```python
from build123d import *

# Parameters (mm, degrees)
BOSS_EXTRUDE6_START     = 1.5
BOSS_EXTRUDE6_DEPTH     = 1.5
BOSS_EXTRUDE7_START     = 3
SKETCH1_5_W             = 11.9
SKETCH1_5_H             = 5.3
SKETCH1_5_W_2           = 1.5
SKETCH1_5_H_2           = 5.936611654
BOSS_EXTRUDE7_DEPTH     = 7.93
BOSS_EXTRUDE8_START     = 10.93
BOSS_EXTRUDE8_OUTLINE_W = 11.9
BOSS_EXTRUDE8_OUTLINE_H = 12.736611654
BOSS_EXTRUDE8_DEPTH     = 0.75
SKETCH4_R               = 1.5
BOSS_EXTRUDE10_DEPTH    = 2.5


# Read off the part's stored shape, not the designer's step: Boss-Extrude8
with BuildPart() as part:
    # Sketch1 → Boss-Extrude6 (new body)
    with BuildSketch(Plane.ZY.offset(94.76563723).offset(BOSS_EXTRUDE6_START)):
        with BuildLine():
            Line((-51.759425025, -53.863488773), (-52.289755114, -53.333158684))
            ThreePointArc((-52.289755114, -53.333158684), (-52.343100233, -53.254101332), (-52.362978418, -53.160824194))
            Line((-52.362978418, -53.160824194), (-52.362978418, -48.300100424))
            Line((-52.362978418, -48.300100424), (-54.862978418, -48.300100424))
            Line((-54.862978418, -48.300100424), (-54.862978418, -61.036712078))
            Line((-54.862978418, -61.036712078), (-42.962978418, -61.036712078))
            Line((-42.962978418, -61.036712078), (-42.962978418, -48.300100424))
            Line((-42.962978418, -48.300100424), (-45.462978418, -48.300100424))
            Line((-45.462978418, -48.300100424), (-45.462978418, -53.156381989))
            ThreePointArc((-45.462978418, -53.156381989), (-45.482008535, -53.252052847), (-45.536201723, -53.333158684))
            Line((-45.536201723, -53.333158684), (-46.066531809, -53.86348877))
            ThreePointArc((-46.066531809, -53.86348877), (-46.147637646, -53.917681958), (-46.243308504, -53.936712075))
            Line((-46.243308504, -53.936712075), (-51.582648329, -53.936712078))
            ThreePointArc((-51.582648329, -53.936712078), (-51.678319187, -53.917681961), (-51.759425025, -53.863488773))
        make_face()
    extrude(amount=BOSS_EXTRUDE6_DEPTH)

    # Sketch1<5> → Boss-Extrude7 (add)
    with BuildSketch(Plane.ZY.offset(94.76563723).offset(BOSS_EXTRUDE7_START)):
        with Locations((-48.912978418, -58.386712078)):
            Rectangle(SKETCH1_5_W, SKETCH1_5_H)
        Polygon((-53.362978418, -55.636712078), (-53.362978418, -54.236712078), (-54.862978418, -54.236712078), (-54.862978418, -55.736712078), (-42.962978418, -55.736712078), (-42.962978418, -54.236712078), (-44.462978418, -54.236712078), (-44.462978418, -55.636712078), align=None)
        with Locations((-54.112978418, -51.268406251)):
            Rectangle(SKETCH1_5_W_2, SKETCH1_5_H_2)
        with Locations((-43.712978418, -51.268406251)):
            Rectangle(SKETCH1_5_W_2, SKETCH1_5_H_2)
    extrude(amount=BOSS_EXTRUDE7_DEPTH)

    # Boss-Extrude8 outline → Boss-Extrude8 (add)
    with BuildSketch(Plane.ZY.offset(94.76563723).offset(BOSS_EXTRUDE8_START)):
        with Locations((-48.912978418, -54.668406251)):
            Rectangle(BOSS_EXTRUDE8_OUTLINE_W, BOSS_EXTRUDE8_OUTLINE_H)
    extrude(amount=BOSS_EXTRUDE8_DEPTH)

    # Sketch4 → Boss-Extrude10 (add)
    # profile 1 of 2: a face of its own
    with BuildSketch(Plane.XZ.offset(61.036712078)):
        with BuildLine():
            Line((-102.26563723, -39.962978418), (-102.26563723, -42.962978418))
            Line((-102.26563723, -42.962978418), (-96.26563723, -42.962978418))
            Line((-96.26563723, -42.962978418), (-96.26563723, -39.962978418))
            ThreePointArc((-96.26563723, -39.962978418), (-99.26563723, -36.962978418), (-102.26563723, -39.962978418))
        make_face()
        with Locations(Location((-99.26563723, -39.962978418, 0), (0, 0, 270))):
            Circle(SKETCH4_R, mode=Mode.SUBTRACT)
    # profile 2 of 2: a face of its own
    with BuildSketch(Plane.XZ.offset(61.036712078)):
        with BuildLine():
            Line((-96.26563723, -57.862978418), (-96.26563723, -54.862978418))
            Line((-96.26563723, -54.862978418), (-102.26563723, -54.862978418))
            Line((-102.26563723, -54.862978418), (-102.26563723, -57.862978418))
            ThreePointArc((-102.26563723, -57.862978418), (-99.26563723, -60.862978418), (-96.26563723, -57.862978418))
        make_face()
        with Locations(Location((-99.26563723, -57.862978418, 0), (0, 0, 270))):
            Circle(SKETCH4_R, mode=Mode.SUBTRACT)
    extrude(amount=-BOSS_EXTRUDE10_DEPTH)


solid = part.part
```
For this review, take the finished solid that the model builds, in its own axes (mm). A direction names the side the tool comes from. Give positions to 0.01 mm unless a question says otherwise; leave off trailing zeros. Write each loop counter-clockwise with the first axis right and the second up, starting at its lowest first coordinate (ties: lowest second). Pieces come first, ordered by that corner, then holes.
Item 1: Take a section at B-B (x = -103.75). Give the boundary of the cut face in (y, z), and give its area (3 significant figures).
Item 2: Insertion check: P1, Ø2, axis at x = -101, y = -51.5, coming from the -Z side; P2, Ø3.5, axis at x = -100, y = -51.5, coming from the +Z side; P3, Ø1.6, axis at x = -97, z = -49, coming from the +Y side; P4, Ø1.8, axis at x = -99.27, z = -57.86, coming from the +Y side. Each pin has a flat end and moves straight along its axis. Give the tip position at first contact, or say it passes through.
Item 3: Wall thickness on probe 1 along Z at (x, y) = (-102.25, -54); probe 2 along X at (y, z) = (-49.25, -45.25); probe 3 along Y at (x, z) = (-101.5, -50.25): over which ranges is each line inside the solid? List them lowest first.
Item 4: Take a section at D-D (z = -59). Give the boundary of the cut face in (x, y), and give its area (3 significant figures).
Item 5: Take a section at C-C (y = -55). Give the boundary of the cut face in (x, z), and give its area (3 significant figures).
Item 6: The part is to be moulded in two halves that separate along X. For faces 1 (the face through (-101, -55, -42.963)), 2 (the face through (-99.84, -59.8, -41.35)), 3 (the face through (-106.446, -55, -49)), say which applies: +X half, -X half, draft (parallel to the pull), parting line (faces both ways), or undercut.
Item 7: Take a section at A-A (z = -48). Give the boundary of the cut face in (x, y).
Item 8: Machinability: for faces 4 (the face through (-102.266, -60, -41)), 5 (the face through (-102, -52, -53.363)), 6 (the face through (-97, -51, -52.363)), 7 (the face through (-100, -58.537, -56)), which of the approach directions +Z, -Z, +X, -X, +Y, -Y give a long, thin tool a straight path to every point of the face, cutting with its end or side? Answer none if there is none.
Established:
1. outline: (-61.04, -54.86) - (-48.3, -54.86) - (-48.3, -53.36) - (-55.64, -53.36) - (-55.64, -44.46) - (-48.3, -44.46) - (-48.3, -42.96) - (-61.04, -42.96) - close
1. area: 86.3 mm2
2. P1: stops at z = -54.86
2. P2: stops at z = -42.96
2. P3: stops at y = -53.94
2. P4: passes through
3. probe 1: z = -54.86 to -53.36, -44.46 to -42.96
3. probe 2: x = -106.45 to -105.7, -97.77 to -96.27
3. probe 3: y = -61.04 to -55.64
4. outline: (-102.04, -61.04) - (-100.24, -61.04) - (-100.24, -58.54) - (-102.04, -58.54) - close; (-98.29, -61.04) - (-96.49, -61.04) - (-96.49, -58.54) - (-98.29, -58.54) - close
4. area: 8.99 mm2
5. outline: (-106.45, -54.86) - (-96.27, -54.86) - (-96.27, -42.96) - (-106.45, -42.96) - close; hole (-105.7, -53.36) - (-97.77, -53.36) - (-97.77, -44.46) - (-105.7, -44.46) - close
5. area: 50.6 mm2
6. face 1: draft
6. face 2: undercut
6. face 3: -X half
7. outline: (-106.45, -61.04) - (-96.27, -61.04) - (-96.27, -53.94) - (-97.77, -53.94) - (-97.77, -55.64) - (-105.7, -55.64) - (-105.7, -48.3) - (-106.45, -48.3) - close
8. face 4: +Z, -X, +Y, -Y
8. face 5: +Y
8. face 6: +X, +Y
8. face 7: -Z, +X, -X, +Y
